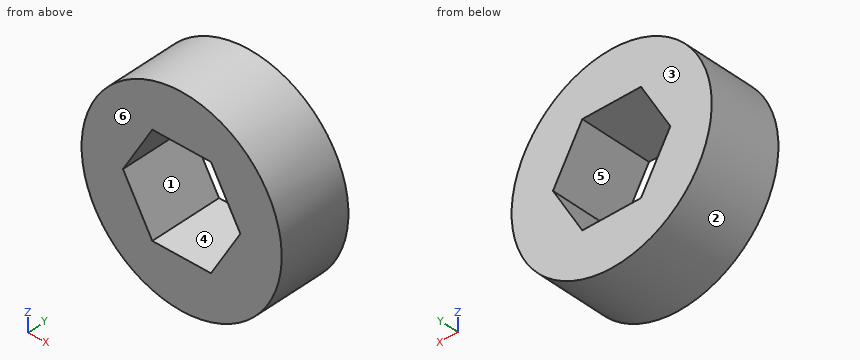
from build123d import *

# Parameters (mm, degrees)
CROQUIS1_R              = 12.5
SALIENTE_EXTRUIR1_DEPTH = 9


with BuildPart() as part:
    # Croquis1 → Saliente-Extruir1 (new body)
    with BuildSketch(Plane(origin=(0, 0, 0), x_dir=(1, 0, 0), z_dir=(0, 1, 0))):
        with Locations(Location((0, 0, 0), (0, 0, 270))):
            Circle(CROQUIS1_R)
        Polygon((7.332348419, 0), (3.666174209, 6.35), (-3.666174209, 6.35), (-7.332348419, 0), (-3.666174209, -6.35), (3.666174209, -6.35), align=None, mode=Mode.SUBTRACT)
    extrude(amount=SALIENTE_EXTRUIR1_DEPTH)


solid = part.part
Design review of the part built by this model. Coordinates are the model's own, in mm. Face numbers are marked on the shaded views. A direction names the side the tool comes from. Round coordinates to 2 decimals unless told otherwise and drop trailing zeros. Loops run counter-clockwise (first coordinate to the right, second up) from the corner with the lowest first, then second, coordinate; pieces in that order, holes last. Notation, with made-up numbers: (83, 89.5) -> (99, 89.5) arc R24 cw to (99, 128.5) -> close; hole circle Ø1 at (-34, 0.25). An arc over 180 degrees is marked (long way). Use one line per item in the form item = value. Start each with the question number.
Q1. We need section A-A on x = 0. Give the boundary of the cut face in (y, z), then the cut area to 3 significant figures.
Q2. Wall thickness on line 1 along X through (y, z) = (5.5, -2); line 2 along X through (y, z) = (2.75, -3); line 3 along Z through (x, y) = (-5.5, 0.5): over which ranges is each line inside the solid? List them lowest first. Write a range as [from, to].
Q3. We need section D-D on x = 9.75. Give the boundary of the cut face in (y, z).
Q4. We need section C-C on z = -5.75. Give the boundary of the cut face in (x, y), then the cut area to 3 significant figures.
Q5. Machinability: for the marked faces 5 and 6, which of the approach directions +Z, -Z, +X, -X, +Y, -Y give a long, thin tool a straight path to every point of the face, cutting with its end or side? Answer none if there is none.
Q6. Draft analysis for pull direction Z (two halves, no side actions). For the marked faces 1, 2, 3 and 4, state which applies: +Z half, -Z half, draft (parallel to the pull), parting line (faces both ways), or undercut.
Q7. For pin 1 Ø3 at (y, z) = (6, -9.5) entering from -X; pin 2 Ø3 at (y, z) = (5.5, -4) entering from +X; pin 3 Ø2 at (y, z) = (6.5, 1.5) entering from -X; pin 4 Ø1 at (x, z) = (-4, -1.5) entering from +Y, all flat-tipped, find the tip position at first contact; note any pin that passes through.
Q8. We need section B-B on y = 7.5. Give the boundary of the cut face in (x, z).
Calculated:
q1.outline = (0, -12.5) -> (9, -12.5) -> (9, -6.35) -> (0, -6.35) -> close; (0, 6.35) -> (9, 6.35) -> (9, 12.5) -> (0, 12.5) -> close
q1.area = 111 mm²
q2.line_1 = [-12.34, -6.18], [6.18, 12.34]
q2.line_2 = [-12.13, -5.6], [5.6, 12.13]
q2.line_3 = [-11.22, -3.17], [3.17, 11.22]
q3.outline = (0, -7.82) -> (9, -7.82) -> (9, 7.82) -> (0, 7.82) -> close
q4.outline = (-11.1, 0) -> (-4.01, 0) -> (-4.01, 9) -> (-11.1, 9) -> close; (4.01, 0) -> (11.1, 0) -> (11.1, 9) -> (4.01, 9) -> close
q4.area = 128 mm²
q5.face_5 = +Y, -Y
q5.face_6 = +Z, -Z, +X, -X, -Y
q6.face_1 = undercut
q6.face_2 = parting line
q6.face_3 = draft
q6.face_4 = undercut
q7.pin_1 = -9.6
q7.pin_2 = 12.25
q7.pin_3 = -12.49
q7.pin_4 = through
q8.outline = circle Ø25 at (0, 0); hole (-7.33, 0) -> (-3.67, -6.35) -> (3.67, -6.35) -> (7.33, 0) -> (3.67, 6.35) -> (-3.67, 6.35) -> close
